Can you work these out from the drawing? Everything is in mm from the part's minimum corner. Round coordinates to 2 decimals unless told otherwise and drop trailing zeros. Write each loop counter-clockwise with the first axis right and the second up, starting at its lowest first coordinate (ties: lowest second). Pieces come first, ordered by that corner, then holes. Notation, with made-up numbers: M 85,63 L 125,63 A10 cw 125,72 Z; hole C 74.5,-11 d2. An arc over 180 degrees is marked long. Answer in a Markdown table with one row per item. Add a question column.
(1) I'm going to push a flat-ended pin straight in: pin 1 (4 mm diameter, centred on x = 20, y = 5, fed in from -Z). Where does the tip first touch, or does it pass through?
(2) Suppose I cut it at B-B, the plane z = 2.5. Write out the boundary of the cut face in (x, y), then the cut area to 3 significant figures.
(3) Suppose I cut it at A-A, the plane y = 5. Write out the boundary of the cut face in (x, z), then the cut area to 3 significant figures.
(4) If I drill on probe 1 along Y at (x, z) = (20, 0.7); probe 2 along X at (y, z) = (4.5, 2.7); probe 3 along X at (y, z) = (4, 2.2), over which ranges is the centre line in solid material (lowest first)?
(5) Suppose I cut it at C-C, the plane x = 23. Write out the boundary of the cut face in (y, z), then the cut area to 3 significant figures.
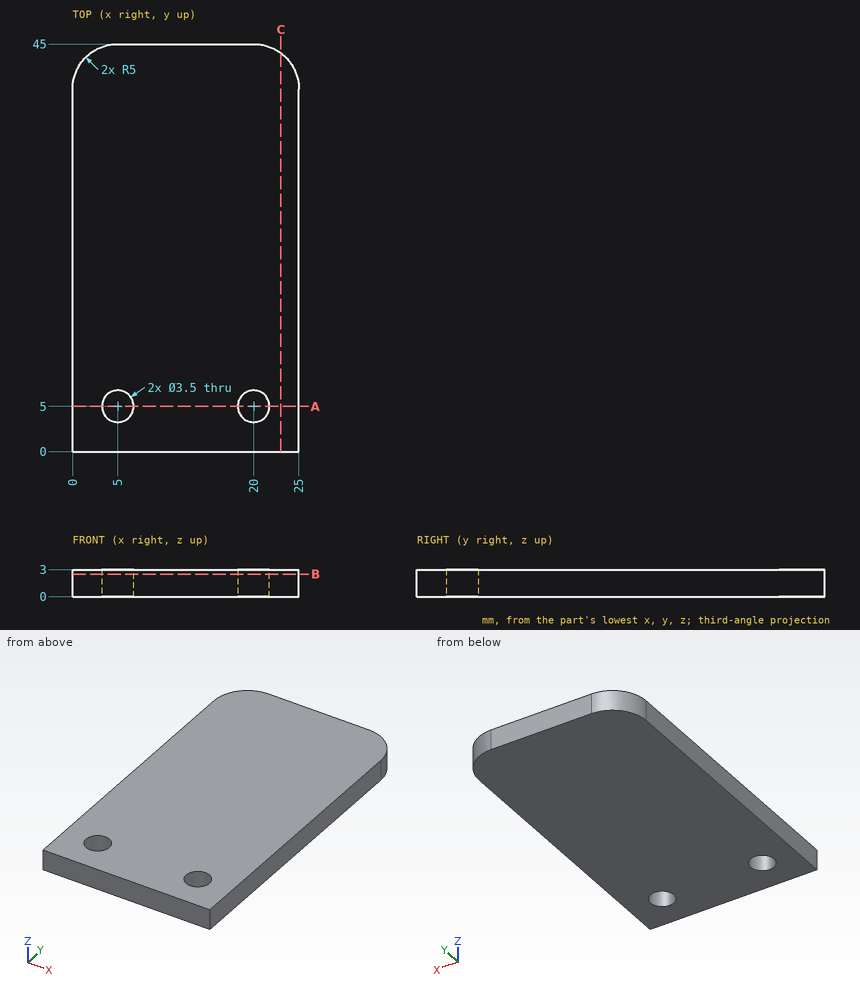
Calculated:
| question | item | result |
|---|---|---|
| 1 | pin 1 | z = 0 |
| 2 | outline | M 0,0 L 25,0 L 25,40 A5 ccw 20,45 L 5,45 A5 ccw 0,40 Z; hole C 5,5 d3.5; hole C 20,5 d3.5 |
| 2 | area | 1,100 mm² |
| 3 | outline | M 0,0 L 3.25,0 L 3.25,3 L 0,3 Z; M 6.75,0 L 18.25,0 L 18.25,3 L 6.75,3 Z; M 21.75,0 L 25,0 L 25,3 L 21.75,3 Z |
| 3 | area | 54.0 mm² |
| 4 | probe 1 | 0 to 3.25, 6.75 to 45 |
| 4 | probe 2 | 0 to 3.32, 6.68 to 18.32, 21.68 to 25 |
| 4 | probe 3 | 0 to 3.56, 6.44 to 18.56, 21.44 to 25 |
| 5 | outline | M 0,0 L 44,0 L 44,3 L 0,3 Z |
| 5 | area | 132 mm² |
